```python
from build123d import *

# Parameters (mm, degrees)
F1_W     = 63
F1_H     = 53
F1_R     = 1.5
F1_R_2   = 1
F1_W_2   = 4
F1_H_2   = 10.5
F2_DEPTH = 1
F3_R     = 2
F4_DEPTH = 25
F5_DEPTH = 25
F6_DEPTH = 25
F7_DEPTH = 20


with BuildPart() as f2:
    # F1 (on face) → F2 (new body)
    with BuildSketch(Plane.XY):
        with Locations((-39.7031286434, 26.5)):
            Rectangle(F1_W, F1_H)
        with Locations((-11.7031286434, 3.5)):
            Circle(F1_R, mode=Mode.SUBTRACT)
        with Locations((-18.2031286434, 7)):
            Circle(F1_R_2, mode=Mode.SUBTRACT)
        with Locations((-18.2031286434, 15)):
            Circle(F1_R_2, mode=Mode.SUBTRACT)
        with Locations((-67.7031286434, 26.5)):
            Circle(F1_R, mode=Mode.SUBTRACT)
        with Locations((-62.2031286434, 36.25)):
            Rectangle(F1_W_2, F1_H_2, mode=Mode.SUBTRACT)
        with BuildLine():
            ThreePointArc((-38.5332978681, 45.6221886318), (-37.9227267856, 44.9111362273), (-37.7031286434, 44))
            ThreePointArc((-37.7031286434, 44), (-40.6142648707, 42.2195981422), (-40.8729594187, 45.6221886318))
            Line((-40.8729594187, 45.6221886318), (-40.8729594187, 50.1384101469))
            Line((-40.8729594187, 50.1384101469), (-38.5332978681, 50.1384101469))
            Line((-38.5332978681, 50.1384101469), (-38.5332978681, 45.6221886318))
        make_face(mode=Mode.SUBTRACT)
        with Locations((-11.7031286434, 49.5)):
            Circle(F1_R, mode=Mode.SUBTRACT)
    extrude(amount=F2_DEPTH)

    # F3
    f3_edges = [f2.edges().sort_by_distance(p)[0] for p in [
        (-71.203129, 53, 0.5),
        (-71.203129, 0, 0.5),
        (-8.203129, 0, 0.5),
        (-8.203129, 53, 0.5),
    ]]
    fillet(f3_edges, radius=F3_R)

    # F1 (on face) → F4 (join)
    with BuildSketch(Plane.XY):
        with Locations((-11.7031286434, 49.5)):
            Circle(F1_R)
        with Locations((-11.7031286434, 3.5)):
            Circle(F1_R)
        with Locations((-67.7031286434, 26.5)):
            Circle(F1_R)
        with Locations((-62.2031286434, 36.25)):
            Rectangle(F1_W_2, F1_H_2)
        with Locations((-18.2031286434, 7)):
            Circle(F1_R_2)
        with Locations((-18.2031286434, 15)):
            Circle(F1_R_2)
        with BuildLine():
            ThreePointArc((-40.8729594187, 45.6221886318), (-40.6142648707, 42.2195981422), (-37.7031286434, 44))
            ThreePointArc((-37.7031286434, 44), (-37.9227267856, 44.9111362273), (-38.5332978681, 45.6221886318))
            Line((-38.5332978681, 45.6221886318), (-40.8729594187, 45.6221886318))
        make_face()
        with BuildLine():
            Line((-40.8729594187, 45.6221886318), (-38.5332978681, 45.6221886318))
            ThreePointArc((-38.5332978681, 45.6221886318), (-39.7031286434, 46), (-40.8729594187, 45.6221886318))
        make_face()
        with BuildLine():
            ThreePointArc((-40.8729594187, 45.6221886318), (-39.7031286434, 46), (-38.5332978681, 45.6221886318))
            Line((-38.5332978681, 45.6221886318), (-38.5332978681, 50.1384101469))
            Line((-38.5332978681, 50.1384101469), (-40.8729594187, 50.1384101469))
            Line((-40.8729594187, 50.1384101469), (-40.8729594187, 45.6221886318))
        make_face()
    extrude(amount=F4_DEPTH)

    # F5 (cut): a face of the model
    f5_faces = [f2.faces().sort_by_distance(p)[0] for p in [
        (-62.2031286434, 36.25, 25),
    ]]
    extrude(f5_faces, amount=-F5_DEPTH, mode=Mode.SUBTRACT)

    # F6 (cut): faces of the model
    f6_faces = [f2.faces().sort_by_distance(p)[0] for p in [
        (-39.7031286434, 45.772355973, 25),
        (-18.2031286434, 15, 25),
        (-18.2031286434, 7, 25),
    ]]
    extrude(f6_faces, amount=-F6_DEPTH, mode=Mode.SUBTRACT)

    # F7 (cut): faces of the model
    f7_faces = [f2.faces().sort_by_distance(p)[0] for p in [
        (-11.7031286434, 49.5, 25),
        (-67.7031286434, 26.5, 25),
        (-11.7031286434, 3.5, 25),
    ]]
    extrude(f7_faces, amount=-F7_DEPTH, mode=Mode.SUBTRACT)


solid = f2.part
```
Build history of the part. All positions in model axes, mm. A direction names the side the tool comes from. Coordinates: 2 decimals unless noted, no trailing zeros. Order: outer loops, then holes, each group sorted by start corner. A loop starts at its lowest first (then second) coordinate and runs counter-clockwise, first axis right, second up.
Item 1: Mould opens along Y. For faces 1 (the cylindrical face through (-10.272, 3.951, 2.972)), 2 (the cylindrical face through (-8.805, 52.43, 0.507)), 3 (the cylindrical face through (-18.94, 7.676, 0.507)), 4 (the cylindrical face through (-68.81, 27.51, 2.97)) say: released by +Y, released by -Y, zero draft, split by the parting line, or undercut.
Filled in:
face 1: undercut
face 2: released by +Y
face 3: undercut
face 4: split by the parting line
Item 2: Saw through at C-C on z = 2.55. List the corners of the cut face in (x, y), then the cut area to 3 significant figures.
Filled in:
outline: circle Ø3 at (-67.7, 26.5); circle Ø3 at (-11.7, 3.5); circle Ø3 at (-11.7, 49.5)
area: 21.2 mm2
Item 3: Tool access for faces 5 (the cylindrical face through (-11.01, 48.17, 2.97)), 6 (the cylindrical face through (-70.63, 52.4, 0.51)): list every direction of +Z, -Z, +X, -X, +Y, -Y with a clear straight run to the whole face (end or side of a thin tool).
Filled in:
face 5: +Z
face 6: +Z, -Z, -X, +Y
Item 4: Saw through at A-A on x = -62.5. List the corners of the cut face in (y, z).
Filled in:
outline: (0, 0) - (31, 0) - (31, 1) - (0, 1) - close; (41.5, 0) - (53, 0) - (53, 1) - (41.5, 1) - close
Item 5: Drop flat-ended pins along their axis: pin 1 Ø5 at (x, y) = (-48.5, 12.5) entering from +Z; pin 2 Ø3.5 at (x, y) = (-39.7, 44) entering from -Z. Give the stop position or say it passes through.
Filled in:
pin 1: stops at z = 1
pin 2: passes through
Item 6: Saw through at B-B on y = 34. List the corners of the cut face in (x, z).
Filled in:
outline: (-71.2, 0) - (-64.2, 0) - (-64.2, 1) - (-71.2, 1) - close; (-60.2, 0) - (-8.2, 0) - (-8.2, 1) - (-60.2, 1) - close
Item 7: Saw through at D-D on x = -34. List the corners of the cut face in (y, z).
Filled in:
outline: (0, 0) - (53, 0) - (53, 1) - (0, 1) - close
Item 8: Drill centre lines: L1, parallel to X at y = 44, z = 0.8; L2, parallel to Z at x = -68, y = 29; L3, parallel to X at y = 49, z = 3.9. Where is each one in solid material? Low to high.
Filled in:
L1: x = -71.2 to -41.7, -37.7 to -8.2
L2: z = 0 to 1
L3: x = -13.12 to -10.29
